Check sheet for the modelled part. Datum: model origin and axes. Units: mm. A direction names the side the tool comes from. Give positions to 0.01 mm unless a question says otherwise; leave off trailing zeros. Write each loop counter-clockwise with the first axis right and the second up, starting at its lowest first coordinate (ties: lowest second). Pieces come first, ordered by that corner, then holes. Notation, with made-up numbers: M 85.25,8.25 L 142.25,8.25 A12 cw 142.25,30.25 Z; hole C 11.5,69.5 d5. An arc over 180 degrees is marked long. One line per item, written item: value. Start each with the question number.
from build123d import *

# Parameters (mm, degrees)
BOSS_EXTRUDE1_DEPTH = 88.3
SKETCH6_R           = 1.65
BOSS_EXTRUDE2_DEPTH = 8.5
CUT_EXTRUDE1_DEPTH  = 93.261259475
SKETCH8_W           = 61.3
SKETCH8_H           = 21.483950942
CUT_EXTRUDE2_DEPTH  = 93.163658782
SKETCH9_W           = 61.3
SKETCH9_H           = 11.699409457
CUT_EXTRUDE3_DEPTH  = 93.53707735
SKETCH10_R          = 1.65
CUT_EXTRUDE4_DEPTH  = 94.043055829
CHAMFER1_SIZE       = 8
CHAMFER1_SIZE2      = 3
CUT_EXTRUDE5_DEPTH  = 93.537077445
FILLET1_R           = 2
CUT_EXTRUDE7_START  = -5.05
CUT_EXTRUDE7_DEPTH  = 5.05
CUT_EXTRUDE8_DEPTH  = 2.5
CHAMFER2_SIZE       = 0.5


with BuildPart() as part:
    # Sketch1 → Boss-Extrude1 (new body)
    with BuildSketch(Plane.ZY):
        with BuildLine():
            Line((-9.5, 8.25), (-9.5, -8.25))
            Line((-9.5, -8.25), (0, -8.25))
            ThreePointArc((0, -8.25), (8.25, 0), (0, 8.25))
            Line((0, 8.25), (-9.5, 8.25))
        make_face()
    extrude(amount=BOSS_EXTRUDE1_DEPTH)

    # Sketch6 → Boss-Extrude2 (add)
    with BuildSketch(Plane(origin=(0, 0, -9.5), x_dir=(-1, 0, 0), z_dir=(0, 0, -1))):
        with BuildLine():
            Line((17.15, -8.25), (17.15, 20))
            ThreePointArc((17.15, 20), (20.99096395, 24.863808737), (26.612654174, 22.254931867))
            Line((26.612654174, 22.254931867), (32.579554775, 10.446054507))
            ThreePointArc((32.579554775, 10.446054507), (34.053942202, 8.842964487), (36.149678114, 8.25))
            Line((36.149678114, 8.25), (52.150321886, 8.25))
            ThreePointArc((52.150321886, 8.25), (54.246057798, 8.842964487), (55.720445225, 10.446054507))
            Line((55.720445225, 10.446054507), (61.687345826, 22.254931867))
            ThreePointArc((61.687345826, 22.254931867), (67.30903605, 24.863808737), (71.15, 20))
            Line((71.15, 20), (71.15, -8.25))
            Line((71.15, -8.25), (17.15, -8.25))
        make_face()
        with Locations((22.15, 20)):
            Circle(SKETCH6_R, mode=Mode.SUBTRACT)
        with Locations(Location((66.15, 20, 0), (0, 0, 180))):
            Circle(SKETCH6_R, mode=Mode.SUBTRACT)
    extrude(amount=-BOSS_EXTRUDE2_DEPTH)

    # Sketch7 → Cut-Extrude1 (cut, through all)
    with BuildSketch(Plane.ZY.offset(88.3)):
        with BuildLine():
            Line((13.481907846, 13.481907846), (4.277996026, 4.277996026))
            ThreePointArc((4.277996026, 4.277996026), (-6.05, 0), (4.277996026, -4.277996026))
            Line((4.277996026, -4.277996026), (13.481907846, -13.481907846))
            Line((13.481907846, -13.481907846), (13.481907846, 13.481907846))
        make_face()
    extrude(amount=-CUT_EXTRUDE1_DEPTH, mode=Mode.SUBTRACT)

    # Sketch8 → Cut-Extrude2 (cut, through all)
    with BuildSketch(Plane.XY.offset(-1)):
        with Locations((-44.15, -2.491975471)):
            Rectangle(SKETCH8_W, SKETCH8_H)
    extrude(amount=CUT_EXTRUDE2_DEPTH, mode=Mode.SUBTRACT)

    # Sketch9 → Cut-Extrude3 (cut, through all)
    with BuildSketch(Plane(origin=(0, 0, -6.05), x_dir=(-1, 0, 0), z_dir=(0, 0, -1))):
        with Locations((44.15, -5.849704729)):
            Rectangle(SKETCH9_W, SKETCH9_H)
    extrude(amount=-CUT_EXTRUDE3_DEPTH, mode=Mode.SUBTRACT)

    # Sketch10 → Cut-Extrude4 (cut, through all)
    with BuildSketch(Plane(origin=(0, 0, -9.5), x_dir=(-1, 0, 0), z_dir=(0, 0, -1))):
        with Locations((22.15, 7)):
            Circle(SKETCH10_R)
        with Locations((66.15, 7)):
            Circle(SKETCH10_R)
    extrude(amount=-CUT_EXTRUDE4_DEPTH, mode=Mode.SUBTRACT)

    # Chamfer1
    chamfer1_edges = [part.edges().sort_by_distance(p)[0] for p in [
        (-44.15, -8.25, -6.05),
    ]]
    chamfer1_side = [part.faces().sort_by_distance(p)[0] for p in [
        (-44.15, -4.125, -6.05),
    ]]
    chamfer(chamfer1_edges, length=CHAMFER1_SIZE, length2=CHAMFER1_SIZE2, reference=chamfer1_side[0])

    # Sketch11 → Cut-Extrude5 (cut, through all)
    with BuildSketch(Plane(origin=(0, 0, -6.05), x_dir=(-1, 0, 0), z_dir=(0, 0, -1))):
        with BuildLine():
            Line((74.8, -8.25), (47.5958626, -1.828822614))
            ThreePointArc((47.5958626, -1.828822614), (44.15, -1.427659244), (40.7041374, -1.828822614))
            Line((40.7041374, -1.828822614), (13.5, -8.25))
            Line((13.5, -8.25), (13.5, -16.427659244))
            Line((13.5, -16.427659244), (74.8, -16.427659244))
            Line((74.8, -16.427659244), (74.8, -8.25))
        make_face()
    extrude(amount=CUT_EXTRUDE5_DEPTH, mode=Mode.SUBTRACT)

    # Fillet1
    fillet1_edges = [part.edges().sort_by_distance(p)[0] for p in [
        (-17.15, 8.25, -5.25),
        (-71.15, 8.25, -5.25),
    ]]
    fillet(fillet1_edges, radius=FILLET1_R)

    # Sketch13 → Cut-Extrude7 (cut)
    with BuildSketch(Plane.XY.offset(-1).offset(CUT_EXTRUDE7_START)):
        Polygon((-69.05, -2.12397244), (-63.25, -2.12397244), (-63.25, 8.674315781), (-66.15, 10.348631561), (-69.05, 8.674315781), align=None)
        Polygon((-25.05, -2.12397244), (-19.25, -2.12397244), (-19.25, 8.674315781), (-22.15, 10.348631561), (-25.05, 8.674315781), align=None)
    extrude(amount=CUT_EXTRUDE7_DEPTH, mode=Mode.SUBTRACT)

    # Sketch14 → Cut-Extrude8 (cut)
    with BuildSketch(Plane.XY.offset(-1)):
        Polygon((-69, 21.645448267), (-69, 18.354551733), (-66.15, 16.709103466), (-63.3, 18.354551733), (-63.3, 21.645448267), (-66.15, 23.290896534), align=None)
        Polygon((-22.15, 23.290896534), (-25, 21.645448267), (-25, 18.354551733), (-22.15, 16.709103466), (-19.3, 18.354551733), (-19.3, 21.645448267), align=None)
    extrude(amount=-CUT_EXTRUDE8_DEPTH, mode=Mode.SUBTRACT)

    # Chamfer2
    # the kernel refuses this chamfer: 0.5 mm, written as the material it takes off along each edge
    with BuildSketch(Plane(origin=(-88.3, 9.535841494, -9.5), x_dir=(0.9996219169112968, 0, -0.02749587661058574), z_dir=(0, -1, 0))) as chamfer2_piece_1:
        Polygon((CHAMFER2_SIZE * 0.999621916911, CHAMFER2_SIZE * 0.0274958766106), (-CHAMFER2_SIZE * 0.0274958766106, CHAMFER2_SIZE * 0.999621916911), (0, 0), align=None)
    extrude(amount=19.071682988, mode=Mode.SUBTRACT)
    with BuildSketch(Plane(origin=(-22.15, 7, -9.5), x_dir=(-1, 0, 0), z_dir=(0, -1, 0))) as chamfer2_piece_2:
        Polygon((1.65 + CHAMFER2_SIZE, 0), (1.65, -CHAMFER2_SIZE), (1.65, 0), align=None)
    revolve(axis=Axis((-22.15, 7, -9.5), (0, 0, -1)), mode=Mode.SUBTRACT)
    with BuildSketch(Plane(origin=(-66.15, 7, -9.5), x_dir=(-1, 0, 0), z_dir=(0, -1, 0))) as chamfer2_piece_3:
        Polygon((1.65 + CHAMFER2_SIZE, 0), (1.65, -CHAMFER2_SIZE), (1.65, 0), align=None)
    revolve(axis=Axis((-66.15, 7, -9.5), (0, 0, -1)), mode=Mode.SUBTRACT)
    with BuildSketch(Plane(origin=(-36.149678114, 8.25, -9.5), x_dir=(0, -0.9996219169112968, -0.027495876610585647), z_dir=(-1, 0, 0))) as chamfer2_piece_4:
        Polygon((CHAMFER2_SIZE * 0.999621916911, CHAMFER2_SIZE * 0.0274958766106), (-CHAMFER2_SIZE * 0.0274958766106, CHAMFER2_SIZE * 0.999621916911), (0, 0), align=None)
    extrude(amount=16.000643772, mode=Mode.SUBTRACT)
    with BuildSketch(Plane(origin=(1.285841494, -8.25, -9.5), x_dir=(0, 0.9996219169112968, -0.027495876610585647), z_dir=(-1, 0, 0)), Plane(origin=(-73.514158506, -8.25, -9.5), x_dir=(0, 0.9996219169112968, -0.027495876610585647), z_dir=(-1, 0, 0))) as chamfer2_piece_5:
        Polygon((CHAMFER2_SIZE * 0.999621916911, -CHAMFER2_SIZE * 0.0274958766106), (-CHAMFER2_SIZE * 0.0274958766106, -CHAMFER2_SIZE * 0.999621916911), (0, 0), align=None)
    extrude(amount=16.071682988, mode=Mode.SUBTRACT)
    with BuildSketch(Plane(origin=(-76.05145266, -8.545388874, -9.5), x_dir=(-0.22963731849575525, 0.9728878037695274, -0.027495876610585463), z_dir=(0.9732557753191584, 0.22972417332075415, 0)), Plane(origin=(-40.7041374, -1.828822614, -9.5), x_dir=(0.22963731849575528, 0.9728878037695274, -0.027495876610585706), z_dir=(0.9732557753191584, -0.2297241733207542, 0))) as chamfer2_piece_6:
        Polygon((CHAMFER2_SIZE * 0.999621916911, CHAMFER2_SIZE * 0.0274958766106), (-CHAMFER2_SIZE * 0.0274958766106, CHAMFER2_SIZE * 0.999621916911), (0, 0), align=None)
    extrude(amount=29.237524998, mode=Mode.SUBTRACT)
    with BuildSketch(Plane(origin=(-44.15, -16.427659244, -9.5), x_dir=(0.22972417332075398, 0.9732557753191584, 0), z_dir=(0.9732557753191584, -0.22972417332075398, 0))) as chamfer2_piece_7:
        Polygon((15 + CHAMFER2_SIZE, 0), (15, CHAMFER2_SIZE), (15, 0), align=None)
    revolve(axis=Axis((-44.15, -16.427659244, -9.5), (0, 0, 1)), revolution_arc=26.561666454, mode=Mode.SUBTRACT)
    with BuildSketch(Plane(origin=(-71.15, 20, -9.5), x_dir=(0.9996219169112968, 0, -0.02749587661058574), z_dir=(0, -1, 0)), Plane(origin=(-17.15, 10.25, -9.5), x_dir=(-0.9996219169112968, 0, -0.02749587661058555), z_dir=(0, 1, 0))) as chamfer2_piece_8:
        Polygon((CHAMFER2_SIZE * 0.999621916911, CHAMFER2_SIZE * 0.0274958766106), (-CHAMFER2_SIZE * 0.0274958766106, CHAMFER2_SIZE * 0.999621916911), (0, 0), align=None)
    extrude(amount=9.75, mode=Mode.SUBTRACT)
    with BuildSketch(Plane(origin=(1.285841494, 8.25, -9.5), x_dir=(0, -0.9996219169112968, -0.027495876610585647), z_dir=(-1, 0, 0))) as chamfer2_piece_9:
        Polygon((CHAMFER2_SIZE * 0.999621916911, CHAMFER2_SIZE * 0.0274958766106), (-CHAMFER2_SIZE * 0.0274958766106, CHAMFER2_SIZE * 0.999621916911), (0, 0), align=None)
    extrude(amount=16.435841494, mode=Mode.SUBTRACT)
    with BuildSketch(Plane(origin=(-73.15, 10.25, -9.5), x_dir=(0, -1, 0), z_dir=(-1, 0, 0))) as chamfer2_piece_10:
        Polygon((2, CHAMFER2_SIZE), (2 + CHAMFER2_SIZE, 0), (2, 0), align=None)
    revolve(axis=Axis((-73.15, 10.25, -9.5), (0, 0, 1)), revolution_arc=90, mode=Mode.SUBTRACT)
    with BuildSketch(Plane(origin=(-15.15, 10.25, -9.5), x_dir=(-1, 0, 0), z_dir=(0, 1, 0))) as chamfer2_piece_11:
        Polygon((2 + CHAMFER2_SIZE, 0), (2, CHAMFER2_SIZE), (2, 0), align=None)
    revolve(axis=Axis((-15.15, 10.25, -9.5), (0, 0, 1)), revolution_arc=90, mode=Mode.SUBTRACT)
    with BuildSketch(Plane(origin=(-36.149678114, 12.25, -9.5), x_dir=(0.8925308347817242, -0.45098637336824104, 0), z_dir=(0.45098637336824104, 0.8925308347817242, 0))) as chamfer2_piece_12:
        Polygon((4 + CHAMFER2_SIZE, 0), (4, -CHAMFER2_SIZE), (4, 0), align=None)
    revolve(axis=Axis((-36.149678114, 12.25, -9.5), (0, 0, -1)), revolution_arc=63.19301373, mode=Mode.SUBTRACT)
    with BuildSketch(Plane(origin=(-26.612654174, 22.254931867, -9.5), x_dir=(0.8921933839669467, -0.4508158630472358, -0.027495876610585532), z_dir=(-0.45098637336824193, -0.8925308347817238, 0)), Plane(origin=(-55.720445225, 10.446054507, -9.5), x_dir=(-0.8921933839669467, -0.4508158630472356, -0.027495876610585574), z_dir=(-0.45098637336824177, 0.8925308347817239, 0))) as chamfer2_piece_13:
        Polygon((CHAMFER2_SIZE * 0.999621916911, CHAMFER2_SIZE * 0.0274958766106), (-CHAMFER2_SIZE * 0.0274958766106, CHAMFER2_SIZE * 0.999621916911), (0, 0), align=None)
    extrude(amount=13.23077803, mode=Mode.SUBTRACT)
    with BuildSketch(Plane(origin=(-22.15, 20, -9.5), x_dir=(1, 0, 0), z_dir=(0, -1, 0))) as chamfer2_piece_14:
        Polygon((5 - CHAMFER2_SIZE, 0), (5, CHAMFER2_SIZE), (5, 0), align=None)
    revolve(axis=Axis((-22.15, 20, -9.5), (0, 0, 1)), revolution_arc=153.19301373, mode=Mode.SUBTRACT)
    with BuildSketch(Plane(origin=(-52.150321886, 12.25, -9.5), x_dir=(0, -1, 0), z_dir=(1, 0, 0))) as chamfer2_piece_15:
        Polygon((4 + CHAMFER2_SIZE, 0), (4, -CHAMFER2_SIZE), (4, 0), align=None)
    revolve(axis=Axis((-52.150321886, 12.25, -9.5), (0, 0, -1)), revolution_arc=63.19301373, mode=Mode.SUBTRACT)
    with BuildSketch(Plane(origin=(-66.15, 20, -9.5), x_dir=(0.892530834781725, 0.45098637336823943, 0), z_dir=(0.45098637336823943, -0.892530834781725, 0))) as chamfer2_piece_16:
        Polygon((5 - CHAMFER2_SIZE, 0), (5, CHAMFER2_SIZE), (5, 0), align=None)
    revolve(axis=Axis((-66.15, 20, -9.5), (0, 0, 1)), revolution_arc=153.19301373, mode=Mode.SUBTRACT)
    with BuildSketch(Plane(origin=(-22.15, 20, -9.5), x_dir=(-1, 0, 0), z_dir=(0, -1, 0))) as chamfer2_piece_17:
        Polygon((1.65 + CHAMFER2_SIZE, 0), (1.65, -CHAMFER2_SIZE), (1.65, 0), align=None)
    revolve(axis=Axis((-22.15, 20, -9.5), (0, 0, -1)), mode=Mode.SUBTRACT)
    with BuildSketch(Plane(origin=(-66.15, 20, -9.5), x_dir=(1, 0, 0), z_dir=(0, 1, 0))) as chamfer2_piece_18:
        Polygon((1.65 + CHAMFER2_SIZE, 0), (1.65, -CHAMFER2_SIZE), (1.65, 0), align=None)
    revolve(axis=Axis((-66.15, 20, -9.5), (0, 0, -1)), mode=Mode.SUBTRACT)
    with BuildSketch(Plane(origin=(0, 9.535841494, -9.5), x_dir=(-0.9996219169112968, 0, -0.02749587661058563), z_dir=(0, -1, 0))) as chamfer2_piece_19:
        Polygon((CHAMFER2_SIZE * 0.999621916911, -CHAMFER2_SIZE * 0.0274958766106), (-CHAMFER2_SIZE * 0.0274958766106, -CHAMFER2_SIZE * 0.999621916911), (0, 0), align=None)
    extrude(amount=19.071682988, mode=Mode.SUBTRACT)
    with BuildSketch(Plane(origin=(-73.15, 8.25, -9.5), x_dir=(0, 0.027495876610585647, 0.9996219169112968), z_dir=(-1, 0, 0))) as chamfer2_piece_20:
        Polygon((CHAMFER2_SIZE * 0.999621916911, -CHAMFER2_SIZE * 0.0274958766106), (-CHAMFER2_SIZE * 0.0274958766106, -CHAMFER2_SIZE * 0.999621916911), (0, 0), align=None)
    extrude(amount=16.435841494, mode=Mode.SUBTRACT)


solid = part.part
1) Gauge pin test, flat ends, axial feed: pin 1 (0.8 mm diameter, centred on y = 20.5, z = -2.5, fed in from -X); pin 2 (2 mm diameter, centred on x = -21, z = -2.5, fed in from -Y); pin 3 (2.5 mm diameter, centred on y = 4.5, z = -3, fed in from +X); pin 4 (3 mm diameter, centred on y = 20, z = -2, fed in from +X). Record the tip position at first contact, or that the pin passes through.
2) Tool access check on faces 4 (the flat face through (-7, 8.25, -5)), 5 (the flat face through (-74.8, -6, -3)), 6 (the flat face through (-64.745, 17.52, -2.232)), 7 (the conical face through (-54.29, 8.711, -9.135)). Record the directions out of +Z, -Z, +X, -X, +Y, -Y that give a thin tool (end or side, any length) a straight path to the whole face; none if there is none.
3) Cross-section at B-B (x = -81.5). Record the boundary of the cut face in (y, z), plus the area to 3 significant figures.
4) Material ranges on L1, parallel to X at y = 8, z = -3.25; L2, parallel to Y at x = -10.5, z = 0.25; L3, parallel to Y at x = -66.15, z = -5.3, recorded low to high. Write a range as from..to.
5) Draft check along X on faces 1 (the flat face through (-7, -8.25, -5)), 2 (the cylindrical face through (-16.58, 8.85, -5.06)), 3 (the flat face through (-27.23, -4.75, -9.25)). Enter one of: released by +X, released by -X, zero draft, split by the parting line, or undercut.
6) Cross-section at D-D (y = 2.5). Record the boundary of the cut face in (x, z), plus the area to 3 significant figures.
7) Cross-section at C-C (z = -4.75). State how many separate pieces and enclosed holes the cut face has, plus the area to 3 significant figures.
8) Cross-section at A-A (z = 2). Record the boundary of the cut face in (x, y).
Data:
1. pin 1: stops at x = -71.15
1. pin 2: stops at y = 9.11
1. pin 3: stops at x = 0
1. pin 4: stops at x = -17.15
2. face 4: +Z, -Z, +X, +Y
2. face 5: +Z, -Y
2. face 6: +Z
2. face 7: -Z, +Y
3. outline: M -8.25,-9 L -7.75,-9.5 L 7.75,-9.5 L 8.25,-9 L 8.25,0 A8.25 ccw 5.83,5.83 L 4.28,4.28 A6.05 cw long -4.28,4.28 L -5.83,5.83 A8.25 ccw -8.25,0 Z
3. area: 124 mm2
4. L1: x = -88.3..-69.05, -63.25..-25.05, -19.25..0
4. L2: y = -8.25..-6.04, 6.04..8.25
4. L3: y = 10.35..18.35, 21.65..25
5. face 1: zero draft
5. face 2: released by +X
5. face 3: undercut
6. outline: M -88.3,-9 L -87.8,-9.5 L -0.5,-9.5 L 0,-9 L 0,-5.51 L -19.25,-5.51 L -19.25,-6.05 L -25.05,-6.05 L -25.05,-5.51 L -63.25,-5.51 L -63.25,-6.05 L -69.05,-6.05 L -69.05,-5.51 L -88.3,-5.51 Z
6. area: 346 mm2
7. separate pieces: 3
7. enclosed holes: 2
7. area: 837 mm2
8. outline: M -88.3,-8 L -74.8,-8 L -74.8,-5.71 L -88.3,-5.71 Z; M -88.3,5.71 L -74.8,5.71 L -74.8,8 L -88.3,8 Z; M -13.5,-8 L 0,-8 L 0,-5.71 L -13.5,-5.71 Z; M -13.5,5.71 L 0,5.71 L 0,8 L -13.5,8 Z
